Model file for the job. Use its own axes, mm. A direction names the side the tool comes from. Coordinates: 2 decimals unless noted, no trailing zeros. Write each loop counter-clockwise with the first axis right and the second up, starting at its lowest first coordinate (ties: lowest second). Pieces come first, ordered by that corner, then holes. Notation, with made-up numbers: (-10, 35) - (31, 35) arc R19 ccw to (31, 39) - close; hole circle Ø5 at (44.5, -29). An arc over 180 degrees is marked (long way). Put each result on its own line as item: value. Start each with the question number.
1. Saw through at C-C, the plane x = 185. Write the cut outline in (y, z).
2. Saw through at A-A, the plane x = 84. Write the cut outline in (y, z), plus the area to 3 significant figures.
3. Saw through at B-B, the plane z = -87. Write the cut outline in (x, y), plus the area to 3 significant figures.
4. Which spindle directions (+Z, -Z, +X, -X, +Y, -Y) get a long thin tool onto all of the face, cutting with end or side? Do faces 1 (the face through (75.008, 6.595, 1.738)), 2 (the face through (81.45, 15, -90)), 3 (the face through (138.85, 21, -80)). Say none if no direction does.
5. Drop flat-ended pins along their axis: P1, Ø4, axis at x = 71.5, z = -95.5, coming from the -Y side; P2, Ø5, axis at x = 68.6, z = -94.64, coming from the +Y side; P3, Ø12, axis at x = 33, y = 7, coming from the -Z side; P4, Ø7, axis at y = 1.5, z = -47, coming from the +X side. Give the stop position or say it passes through.
6. Drill centre lines: L1, parallel to Y at x = 5.7, z = -78; L2, parallel to X at y = 1, z = -28.5; L3, parallel to X at y = 18.5, z = -83. Where is each one in solid material? Low to high. Write a range as from..to.
7. Pull direction X, two halves, no side cores. Call faces 4 (the face through (81.45, 21, -6)), 5 (the face through (6, 26.35, -80)), 6 (the face through (73.95, 10, -5)): released by +X, released by -X, zero draft, split by the parting line, or undercut.
```python
from build123d import *

# Parameters (mm, degrees)
SKETCH1_W           = 12.7
SKETCH1_H           = 58.9
BOSS_EXTRUDE1_DEPTH = 6.35
SKETCH6_W           = 16.7
SKETCH6_H           = 10
SKETCH6_W_2         = 7
SKETCH6_W_3         = 8.35
BOSS_EXTRUDE5_DEPTH = 20
FILLET6_SIZE        = 8
FILLET6_SIZE_2      = 20
SKETCH7_R           = 1.65
CUT_EXTRUDE1_DEPTH  = 219.058988591
BOSS_EXTRUDE6_DEPTH = 30
SKETCH10_W          = 25.7
SKETCH10_H          = 17.3
CUT_EXTRUDE2_DEPTH  = 229.063149203
SKETCH11_R          = 6.5
SKETCH11_W          = 8.2
SKETCH11_H          = 8.4
BOSS_EXTRUDE7_DEPTH = 2
SKETCH12_R          = 6.5
SKETCH12_W          = 8.2
SKETCH12_H          = 8.4
BOSS_EXTRUDE8_DEPTH = 1.525
SKETCH14_W          = 8.05
SKETCH14_H          = 18
SKETCH14_W_2        = 8.35
SKETCH14_H_2        = 10
CUT_EXTRUDE4_DEPTH  = 230.655188552
CUT_EXTRUDE5_DEPTH  = 230.655188544
SKETCH17_R          = 2
CUT_EXTRUDE6_DEPTH  = 231.096084549
CHAMFER1_SIZE       = 10


with BuildPart() as part:
    # Sketch1 → Boss-Extrude1 (new body)
    with BuildSketch(Plane(origin=(0, 0, 0), x_dir=(1, 0, 0), z_dir=(0, 1, 0))):
        Polygon((0, 101.6), (0, 71.6), (20.5, 71.6), (33.2, 71.6), (95.5, 71.6), (108.2, 71.6), (165.5, 71.6), (178.2, 71.6), (203.2, 71.6), (203.2, 101.6), align=None)
        with Locations((26.85, 42.15)):
            Rectangle(SKETCH1_W, SKETCH1_H)
        with Locations((101.85, 42.15)):
            Rectangle(SKETCH1_W, SKETCH1_H)
        with Locations((171.85, 42.15)):
            Rectangle(SKETCH1_W, SKETCH1_H)
        Polygon((20.5, 12.7), (0, 12.7), (0, 0), (203.2, 0), (203.2, 12.7), (178.2, 12.7), (165.5, 12.7), (108.2, 12.7), (95.5, 12.7), (33.2, 12.7), align=None)
    extrude(amount=BOSS_EXTRUDE1_DEPTH)

    # Sketch6 → Boss-Extrude5 (add)
    with BuildSketch(Plane(origin=(0, 6.35, 0), x_dir=(1, 0, 0), z_dir=(0, 1, 0))):
        with Locations((138.85, 79.6)):
            Rectangle(SKETCH6_W, SKETCH6_H)
        with Locations((191.7, 79.6)):
            Rectangle(SKETCH6_W_2, SKETCH6_H)
        with Locations((134.675, 79.6)):
            Rectangle(SKETCH6_W_3, SKETCH6_H)
        with Locations((86, 79.6)):
            Rectangle(SKETCH6_W_2, SKETCH6_H)
        with Locations((53.7, 79.6)):
            Rectangle(SKETCH6_W_2, SKETCH6_H)
        with Locations((5.7, 79.6)):
            Rectangle(SKETCH6_W_2, SKETCH6_H)
    extrude(amount=BOSS_EXTRUDE5_DEPTH)

    # Fillet6
    # an asymmetric fillet: 20, 8 mm, written as the material it adds along each edge
    with BuildSketch(Plane(origin=(82.5, 6.35, -84.6), x_dir=(-1, 0, 0), z_dir=(0, 0, 1))) as fillet6_piece_1:
        with BuildLine():
            Bezier((FILLET6_SIZE, 0), (0, 0), (0, -FILLET6_SIZE_2), weights=[1, 0.707106781, 1])
            Line((0, -FILLET6_SIZE_2), (-0.4, -20))
            Line((-0.4, -20), (-0.4, 0.4))
            Line((-0.4, 0.4), (8, 0.4))
            Line((8, 0.4), (FILLET6_SIZE, 0))
        make_face()
    extrude(amount=10)
    with BuildSketch(Plane(origin=(89.5, 6.35, -84.6), x_dir=(0, 0, -1), z_dir=(-1, 0, 0))) as fillet6_piece_2:
        with BuildLine():
            Bezier((FILLET6_SIZE, 0), (0, 0), (0, -FILLET6_SIZE_2), weights=[1, 0.707106781, 1])
            Line((0, -FILLET6_SIZE_2), (-0.4, -20))
            Line((-0.4, -20), (-0.4, 0.4))
            Line((-0.4, 0.4), (8, 0.4))
            Line((8, 0.4), (FILLET6_SIZE, 0))
        make_face()
    extrude(amount=7)
    with BuildSketch(Plane(origin=(89.5, 6.35, -84.6), x_dir=(0, 0, -1), z_dir=(-1, 0, 0))) as fillet6_piece_3a_section:
        with BuildLine():
            Bezier((FILLET6_SIZE, 0), (0, 0), (0, -FILLET6_SIZE_2), weights=[1, 0.707106781, 1])
            Line((0, -FILLET6_SIZE_2), (-0.4, -20))
            Line((-0.4, -20), (-0.4, 0.4))
            Line((-0.4, 0.4), (8, 0.4))
            Line((8, 0.4), (FILLET6_SIZE, 0))
        make_face()
    fillet6_piece_3a = extrude(amount=57, mode=Mode.PRIVATE)
    fillet6_piece_3a = split(fillet6_piece_3a, bisect_by=Plane(origin=(82.5, 11.442766382, -86.187108648), z_dir=(-1, 0, 0)), keep=Keep.TOP, mode=Mode.PRIVATE)
    with BuildSketch(Plane(origin=(82.5, 6.35, -134.6), x_dir=(-1, 0, 0), z_dir=(0, 0, 1))) as fillet6_piece_3b_section:
        with BuildLine():
            Bezier((FILLET6_SIZE, 0), (0, 0), (0, -FILLET6_SIZE_2), weights=[1, 0.707106781, 1])
            Line((0, -FILLET6_SIZE_2), (-0.4, -20))
            Line((-0.4, -20), (-0.4, 0.4))
            Line((-0.4, 0.4), (8, 0.4))
            Line((8, 0.4), (FILLET6_SIZE, 0))
        make_face()
    fillet6_piece_3b = extrude(amount=60, mode=Mode.PRIVATE)
    fillet6_piece_3b = split(fillet6_piece_3b, bisect_by=Plane(origin=(80.912890407, 11.442765861, -84.6), z_dir=(0, 0, -1)), keep=Keep.TOP, mode=Mode.PRIVATE)
    fillet6_piece_3 = fillet6_piece_3a & fillet6_piece_3b
    add(fillet6_piece_3)

    # Sketch7 → Cut-Extrude1 (cut, through all)
    with BuildSketch(Plane.XY.offset(-74.6)):
        with Locations((191.7, 21.3)):
            Circle(SKETCH7_R)
        with Locations((191.7, 11.4)):
            Circle(SKETCH7_R)
        with Locations((143.7, 11.4)):
            Circle(SKETCH7_R)
        with Locations((143.7, 21.3)):
            Circle(SKETCH7_R)
        with Locations((86, 21.3)):
            Circle(SKETCH7_R)
        with Locations((86, 11.4)):
            Circle(SKETCH7_R)
        with Locations((134, 21.3)):
            Circle(SKETCH7_R)
        with Locations((134, 11.4)):
            Circle(SKETCH7_R)
        with Locations((5.7, 21.3)):
            Circle(SKETCH7_R)
        with Locations((5.7, 11.4)):
            Circle(SKETCH7_R)
        with Locations((53.7, 11.4)):
            Circle(SKETCH7_R)
        with Locations((53.7, 21.3)):
            Circle(SKETCH7_R)
    extrude(amount=-CUT_EXTRUDE1_DEPTH, mode=Mode.SUBTRACT)

    # Sketch9 → Boss-Extrude6 (add)
    with BuildSketch(Plane(origin=(0, 0, -101.6), x_dir=(-1, 0, 0), z_dir=(0, 0, -1))):
        Polygon((-73.95, 6.35), (-73.95, 14.75), (-65.75, 14.75), (-65.75, 6.35), (-55.75, 6.35), (-55.75, 24.55), (-81.45, 24.55), (-81.45, 6.35), align=None)
    boss_extrude6 = extrude(amount=-BOSS_EXTRUDE6_DEPTH)

    # Mirror1: Boss-Extrude6 across plane
    add(boss_extrude6.mirror(Plane(origin=(0, 0, -50.8), x_dir=(1, 0, 0), z_dir=(0, 0, -1))))

    # Sketch10 → Cut-Extrude2 (cut, through all)
    with BuildSketch(Plane(origin=(0, 6.35, 0), x_dir=(-1, 0, 0), z_dir=(0, -1, 0))):
        with Locations((-68.6, 21.35)):
            Rectangle(SKETCH10_W, SKETCH10_H)
    extrude(amount=-CUT_EXTRUDE2_DEPTH, mode=Mode.SUBTRACT)

    # Sketch11 → Boss-Extrude7 (add)
    with BuildSketch(Plane(origin=(0, 0, -101.6), x_dir=(-1, 0, 0), z_dir=(0, 0, -1))):
        with Locations((-69.85, 10.55)):
            Circle(SKETCH11_R)
        with Locations((-69.85, 10.55)):
            Rectangle(SKETCH11_W, SKETCH11_H, mode=Mode.SUBTRACT)
    boss_extrude7 = extrude(amount=BOSS_EXTRUDE7_DEPTH)

    # Sketch12 → Boss-Extrude8 (add)
    with BuildSketch(Plane(origin=(0, 0, -103.6), x_dir=(-1, 0, 0), z_dir=(0, 0, -1))):
        with Locations((-69.85, 10.55)):
            Circle(SKETCH12_R)
        with Locations((-69.85, 10.55)):
            Rectangle(SKETCH12_W, SKETCH12_H, mode=Mode.SUBTRACT)
    boss_extrude8 = extrude(amount=BOSS_EXTRUDE8_DEPTH)

    # Mirror2: Boss-Extrude7, Boss-Extrude8 across plane
    add(boss_extrude7.mirror(Plane(origin=(0, 0, -50.8), x_dir=(1, 0, 0), z_dir=(0, 0, -1))))
    add(boss_extrude8.mirror(Plane(origin=(0, 0, -50.8), x_dir=(1, 0, 0), z_dir=(0, 0, -1))))

    # Sketch14 → Cut-Extrude4 (cut, through all)
    with BuildSketch(Plane(origin=(0, 6.35, 0), x_dir=(1, 0, 0), z_dir=(0, 1, 0))):
        with Locations((85.475, 83.6)):
            Rectangle(SKETCH14_W, SKETCH14_H)
        with Locations((134.675, 79.6)):
            Rectangle(SKETCH14_W_2, SKETCH14_H_2)
    extrude(amount=CUT_EXTRUDE4_DEPTH, mode=Mode.SUBTRACT)

    # Sketch15 → Cut-Extrude5 (cut, through all)
    with BuildSketch(Plane(origin=(0, 6.35, 0), x_dir=(1, 0, 0), z_dir=(0, 1, 0))):
        Polygon((188.2, 84.6), (195.2, 84.6), (203.2, 84.6), (203.2, 101.6), (81.45, 101.6), (81.45, 84.6), (138.85, 84.6), (147.2, 84.6), align=None)
        Polygon((0, 101.6), (0, 84.6), (57.2, 84.6), (55.75, 84.6), (55.75, 101.6), align=None)
    extrude(amount=-CUT_EXTRUDE5_DEPTH, mode=Mode.SUBTRACT)

    # Sketch17 → Cut-Extrude6 (cut, through all)
    with BuildSketch(Plane(origin=(0, 24.55, 0), x_dir=(1, 0, 0), z_dir=(0, 1, 0))):
        with Locations(Location((68.6, 6.6355, 0), (0, 0, 270))):
            Circle(SKETCH17_R)
        with Locations(Location((68.6, 78.6355, 0), (0, 0, 270))):
            Circle(SKETCH17_R)
        with Locations(Location((68.6, 94.6355, 0), (0, 0, 270))):
            Circle(SKETCH17_R)
    extrude(amount=-CUT_EXTRUDE6_DEPTH, mode=Mode.SUBTRACT)

    # Chamfer1
    # the kernel refuses this chamfer: 10 mm, written as the material it adds along each edge
    with BuildSketch(Plane(origin=(2.2, 6.35, -84.6), x_dir=(-0.9996219169112968, -0.027495876610586386, 0), z_dir=(0, 0, 1))) as chamfer1_piece_1_section:
        Polygon((CHAMFER1_SIZE * 0.999621916911, -CHAMFER1_SIZE * 0.0274958766106), (-CHAMFER1_SIZE * 0.0274958766106, -CHAMFER1_SIZE * 0.999621916911), (0, 0), align=None)
    chamfer1_piece_1 = extrude(amount=10, mode=Mode.PRIVATE)
    chamfer1_piece_1 = split(chamfer1_piece_1, bisect_by=Plane(origin=(0, 10.91513357, -79.6), z_dir=(1, 0, 0)), keep=Keep.TOP, mode=Mode.PRIVATE)
    add(chamfer1_piece_1)
    with BuildSketch(Plane(origin=(81.45, 6.35, -71.6), x_dir=(-0.027495876610586313, 0.9996219169112968, 0), z_dir=(0, 0, -1))) as chamfer1_piece_2:
        Polygon((CHAMFER1_SIZE * 0.999621916911, CHAMFER1_SIZE * 0.0274958766106), (-CHAMFER1_SIZE * 0.0274958766106, CHAMFER1_SIZE * 0.999621916911), (0, 0), align=None)
    extrude(amount=13)
    with BuildSketch(Plane(origin=(81.45, 6.35, 0), x_dir=(0.9996219169112968, -0.027495876610586403, 0), z_dir=(0, 0, -1))) as chamfer1_piece_3:
        Polygon((CHAMFER1_SIZE * 0.999621916911, -CHAMFER1_SIZE * 0.0274958766106), (-CHAMFER1_SIZE * 0.0274958766106, -CHAMFER1_SIZE * 0.999621916911), (0, 0), align=None)
    extrude(amount=12.7)
    with BuildSketch(Plane(origin=(55.75, 6.35, 0), x_dir=(-0.9996219169112968, -0.027495876610586403, 0), z_dir=(0, 0, -1))) as chamfer1_piece_4:
        Polygon((CHAMFER1_SIZE * 0.999621916911, CHAMFER1_SIZE * 0.0274958766106), (-CHAMFER1_SIZE * 0.0274958766106, CHAMFER1_SIZE * 0.999621916911), (0, 0), align=None)
    extrude(amount=12.7)
    with BuildSketch(Plane(origin=(138.85, 6.35, -74.6), x_dir=(-0.9996219169112968, -0.027495876610586365, 0), z_dir=(0, 0, -1))) as chamfer1_piece_5:
        Polygon((CHAMFER1_SIZE * 0.999621916911, CHAMFER1_SIZE * 0.0274958766106), (-CHAMFER1_SIZE * 0.0274958766106, CHAMFER1_SIZE * 0.999621916911), (0, 0), align=None)
    extrude(amount=10)
    with BuildSketch(Plane(origin=(195.2, 6.35, -74.6), x_dir=(0.9996219169112968, -0.027495876610586365, 0), z_dir=(0, 0, -1))) as chamfer1_piece_6_section:
        Polygon((CHAMFER1_SIZE * 0.999621916911, -CHAMFER1_SIZE * 0.0274958766106), (-CHAMFER1_SIZE * 0.0274958766106, -CHAMFER1_SIZE * 0.999621916911), (0, 0), align=None)
    chamfer1_piece_6 = extrude(amount=10, mode=Mode.PRIVATE)
    chamfer1_piece_6 = split(chamfer1_piece_6, bisect_by=Plane(origin=(203.2, 9.807184123, -79.6), z_dir=(-1, 0, 0)), keep=Keep.TOP, mode=Mode.PRIVATE)
    add(chamfer1_piece_6)


solid = part.part
```
Final values:
1. outline: (0, -84.6) - (6.35, -84.6) - (6.35, -71.6) - (0, -71.6) - close; (0, -12.7) - (6.35, -12.7) - (6.35, 0) - (0, 0) - close
2. outline: (0, -84.6) - (13.8, -84.6) - (13.8, -71.6) - (0, -71.6) - close; (0, -12.7) - (13.8, -12.7) - (13.8, 0) - (0, 0) - close
2. area: 355 mm²
3. outline: (55.75, 0) - (81.45, 0) - (81.45, 24.55) - (55.75, 24.55) - close; hole (65.75, 6.35) - (73.95, 6.35) - (73.95, 14.75) - (65.75, 14.75) - close
3. area: 562 mm²
4. face 1: +Z
4. face 2: -Z, +Y
4. face 3: +Z, -Z, +Y
5. P1: stops at y = 0
5. P2: stops at y = 24.55
5. P3: stops at z = -84.6
5. P4: stops at x = 178.2
6. L1: y = 0..9.75, 13.05..19.65, 22.95..26.35
6. L2: x = 20.5..33.2, 95.5..108.2, 165.5..178.2
6. L3: x = 2.2..9.2, 50.2..81.45, 138.85..147.2, 188.2..195.2
7. face 4: released by +X
7. face 5: zero draft
7. face 6: undercut
